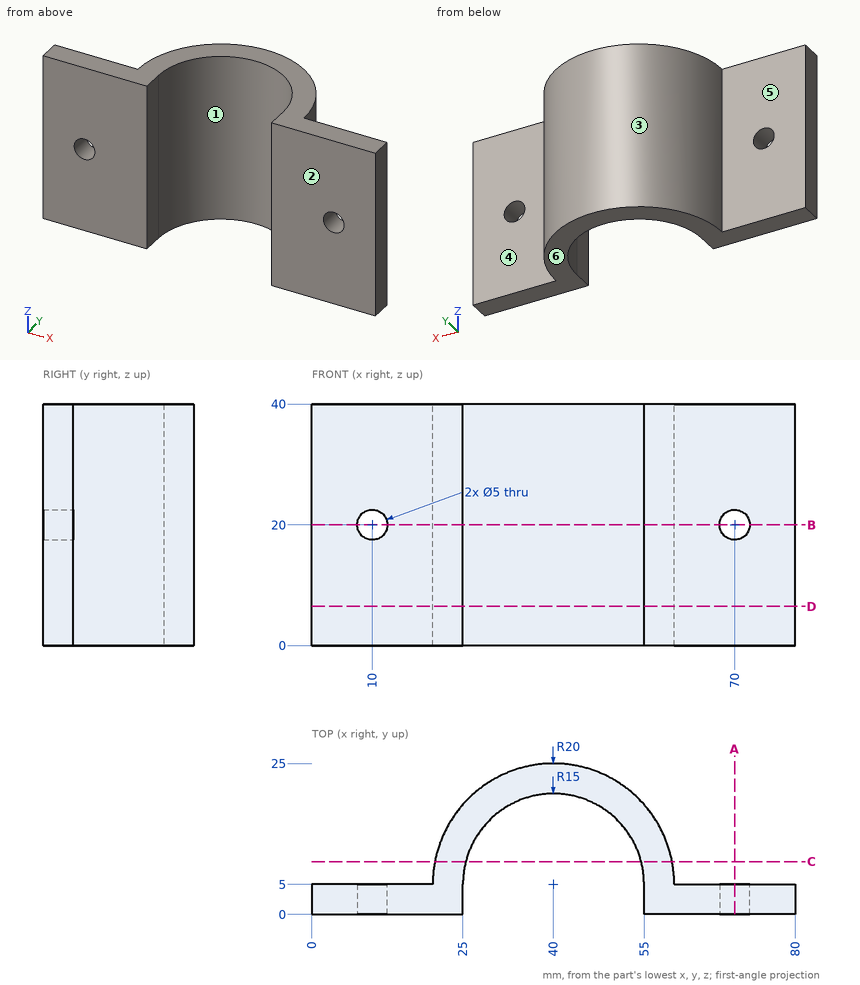
Verification items for this drawing (mm, ordinates from the low corner). A direction names the side the tool comes from. Coordinates: 2 decimals unless noted, no trailing zeros. Order: outer loops, then holes, each group sorted by start corner. A loop starts at its lowest first (then second) coordinate and runs counter-clockwise, first axis right, second up. Notation, with made-up numbers: M 40,18.5 L 75,18.5 A19 ccw 75,33.5 Z; hole C 7.5,1 d6. An arc over 180 degrees is marked long. One line per item, written item: value. Start each with the question number.
Item 1: Sectioned sample at D-D on z = 6.5. Record the cut outline in (x, y).
Item 2: Sectioned sample at B-B on z = 20. Record the cut outline in (x, y).
Item 3: Depth check by flat-ended pin: P1, Ø1, axis at y = 7, z = 13, coming from the -X side; P2, Ø8, axis at y = 22, z = 4.5, coming from the +X side; P3, Ø4, axis at x = 13.5, z = 32, coming from the +Y side; P4, Ø3, axis at x = 10, z = 20, coming from the +Y side. Enter the tip coordinate at first touch or a pass-through.
Item 4: Sectioned sample at A-A on x = 70. Record the cut outline in (y, z), then the cut area to 3 significant figures.
Item 5: Access from +Z, -Z, +X, -X, +Y, -Y to the whole of each face (thin tool, end or side, straight path). Record for the marked faces 4, 5 and 6.
Item 6: Mould release check, pull along X, two halves, no side actions. Record for the marked faces 1, 2 and 3: pulls with the +X half, pulls with the -X half, needs draft (parallel to the pull), parting line crosses it, or undercut.
Item 7: Thickness scan on probe 1 along Z at (x, y) = (70, 3.7); probe 2 along Y at (x, z) = (70.5, 17.5); probe 3 along X at (y, z) = (17, 35.5). Record the ranges inside material, lowest first.
Item 8: Sectioned sample at C-C on y = 8.75. Record the cut outline in (x, z).
Calculated:
1. outline: M 0,0 L 25,0 L 25,5 A15 cw 55,5 L 55,0 L 80,0 L 80,5 L 60,5 A20 ccw 20,5 L 0,5 Z
2. outline: M 0,0 L 7.5,0 L 7.5,5 L 0,5 Z; M 12.5,0 L 25,0 L 25,5 A15 cw 55,5 L 55,0 L 67.5,0 L 67.5,5 L 60,5 A20 ccw 20,5 L 12.5,5 Z; M 72.5,0 L 80,0 L 80,5 L 72.5,5 Z
3. P1: x = 20.06
3. P2: x = 55.2
3. P3: y = 5
3. P4: through
4. outline: M 0,0 L 5,0 L 5,17.5 L 0,17.5 Z; M 0,22.5 L 5,22.5 L 5,40 L 0,40 Z
4. area: 175 mm^2
5. face 4: +Z, -Z, +X, +Y
5. face 5: +Z, -Z, -X, +Y
5. face 6: -Z, +X, -X, +Y, -Y
6. face 1: undercut
6. face 2: needs draft
6. face 3: parting line crosses it
7. probe 1: 0 to 17.5, 22.5 to 40
7. probe 2: 0 to 5
7. probe 3: 24 to 31, 49 to 56
8. outline: M 20.35,0 L 25.48,0 L 25.48,40 L 20.35,40 Z; M 54.52,0 L 59.65,0 L 59.65,40 L 54.52,40 Z
